```python
from build123d import *

# Parameters (mm, degrees)
SKETCH2_W           = 100
SKETCH2_H           = 60
BOSS_EXTRUDE1_DEPTH = 15
SKETCH3_W           = 25
SKETCH3_H           = 15
BOSS_EXTRUDE2_DEPTH = 25
SKETCH4_W           = 25
SKETCH4_H           = 15
BOSS_EXTRUDE3_DEPTH = 25
SKETCH5_W           = 25
SKETCH5_H           = 15
CUT_EXTRUDE1_DEPTH  = 15
SKETCH6_W           = 25
SKETCH6_H           = 15
CUT_EXTRUDE2_DEPTH  = 15


with BuildPart() as part:
    # Sketch2 → Boss-Extrude1 (new body)
    with BuildSketch(Plane(origin=(0, 0, 0), x_dir=(1, 0, 0), z_dir=(0, 1, 0))):
        with Locations((2.681325602, -1.373990244)):
            Rectangle(SKETCH2_W, SKETCH2_H)
    extrude(amount=BOSS_EXTRUDE1_DEPTH)

    # Sketch3 → Boss-Extrude2 (add)
    with BuildSketch(Plane(origin=(0, 15, 0), x_dir=(1, 0, 0), z_dir=(0, 1, 0))):
        with Locations((-34.818674398, 21.126009756)):
            Rectangle(SKETCH3_W, SKETCH3_H)
    extrude(amount=BOSS_EXTRUDE2_DEPTH)

    # Sketch4 → Boss-Extrude3 (add)
    with BuildSketch(Plane(origin=(0, 15, 0), x_dir=(1, 0, 0), z_dir=(0, 1, 0))):
        with Locations((40.181325602, -23.873990244)):
            Rectangle(SKETCH4_W, SKETCH4_H)
    extrude(amount=BOSS_EXTRUDE3_DEPTH)

    # Sketch5 → Cut-Extrude1 (cut)
    with BuildSketch(Plane(origin=(0, 15, 0), x_dir=(1, 0, 0), z_dir=(0, 1, 0))):
        with Locations((-34.818674398, -23.873990244)):
            Rectangle(SKETCH5_W, SKETCH5_H)
    extrude(amount=-CUT_EXTRUDE1_DEPTH, mode=Mode.SUBTRACT)

    # Sketch6 → Cut-Extrude2 (cut)
    with BuildSketch(Plane(origin=(0, 15, 0), x_dir=(1, 0, 0), z_dir=(0, 1, 0))):
        with Locations((40.181325602, 21.126009756)):
            Rectangle(SKETCH6_W, SKETCH6_H)
    extrude(amount=-CUT_EXTRUDE2_DEPTH, mode=Mode.SUBTRACT)


solid = part.part
```
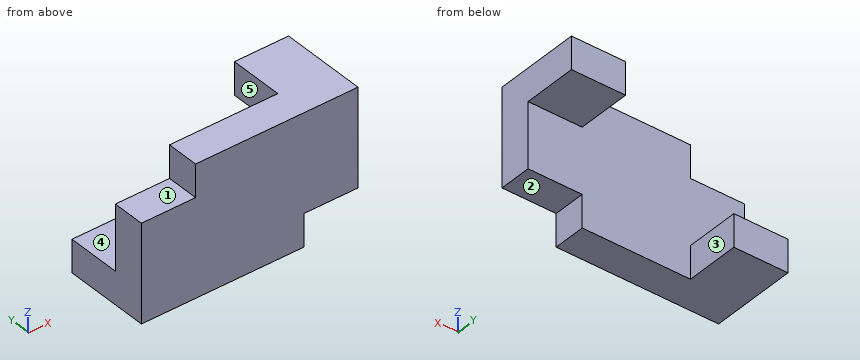
Part model, mm, in its own coordinate system. Face numbers are marked on the shaded views. A direction names the side the tool comes from. Round coordinates to 2 decimals unless told otherwise and drop trailing zeros. Order: outer loops, then holes, each group sorted by start corner. A loop starts at its lowest first (then second) coordinate and runs counter-clockwise, first axis right, second up. Notation, with made-up numbers: M -1.75,59.5 L 43.25,59.5 A21 cw 43.25,76.5 Z; hole C 29,-14 d10. An arc over 180 degrees is marked long. Answer in a Markdown table with one row per item. Add a question column.
Q1. Cut at B-B on z = 23. Give the cut face in (x, y).
Q2. Cut at D-D on x = -29. Give the cut face in (y, z), and give its area (3 significant figures).
Q3. Cut at C-C on y = 10. Give the cut face in (x, z), and give its area (3 significant figures).
Q4. 3-axis set-ups, long thin cutter, end or side, ignore diameter. For the marked faces 1, 2, 3, 4 and 5: which of +Z, -Z, +X, -X, +Y, -Y reach the whole face in a straight line?
Q5. Pin check, flat tips, straight feed: pin 1 (4 mm diameter, centred on x = -20.5, z = -12, fed in from +Y); pin 2 (6 mm diameter, centred on x = -27, y = 4.5, fed in from +Z); pin 3 (4.5 mm diameter, centred on y = 5, z = 26.5, fed in from -X). Stop position of each tip, or through.
Q6. Wall check: L1, parallel to Z at x = 41.5, y = 12.5; L2, parallel to Y at x = -18.5, z = 6; L3, parallel to X at y = 13.5, z = 28. Give the ranges that are in metal, low to high. Write a range as from..to.
Q7. Cut at A-A on y = 21.5. Give the cut face in (x, z), and give its area (3 significant figures).
Established:
| question | item | result |
|---|---|---|
| 1 | outline | M -22.32,0 L 52.68,0 L 52.68,40 L 27.68,40 L 27.68,15 L -22.32,15 Z |
| 2 | outline | M 0,-28.63 L 40,-28.63 L 40,-13.63 L 15,-13.63 L 15,16.37 L 0,16.37 Z |
| 2 | area | 1,050 mm2 |
| 3 | outline | M -47.32,-28.63 L 27.68,-28.63 L 27.68,-13.63 L 52.68,-13.63 L 52.68,31.37 L -22.32,31.37 L -22.32,16.37 L -47.32,16.37 Z |
| 3 | area | 5,250 mm2 |
| 4 | face 1 | +Z, -X, +Y, -Y |
| 4 | face 2 | -Z, +X, +Y, -Y |
| 4 | face 3 | +Z, -Z, +X, +Y |
| 4 | face 4 | +Z, +X, -X, +Y |
| 4 | face 5 | +Z, -Z, -X, +Y |
| 5 | pin 1 | stops at y = 15 |
| 5 | pin 2 | stops at z = 16.37 |
| 5 | pin 3 | stops at x = -22.32 |
| 6 | L1 | z = -13.63..31.37 |
| 6 | L2 | y = 0..15 |
| 6 | L3 | x = -22.32..52.68 |
| 7 | outline | M -47.32,-28.63 L -22.32,-28.63 L -22.32,-13.63 L -47.32,-13.63 Z; M 27.68,16.37 L 52.68,16.37 L 52.68,31.37 L 27.68,31.37 Z |
| 7 | area | 750 mm2 |
